Autodesk Inventor part; units mm, degrees
ref_plane "YZ Plane" through (0, 0, 0) normal (1, 0, 0) x (0, 1, 0)
ref_plane "XZ Plane" through (0, 0, 0) normal (0, 1, 0) x (-1, 0, 0)
ref_plane "XY Plane" through (0, 0, 0) normal (0, 0, 1) x (1, 0, 0)
sketch "Sketch1" plane through (0, 0, 0) normal (0, 0, 1) x (1, 0, 0)
  line L0 (-34.8609, 0) -> (34.8609, 0) construction
  line L1 (0, -34.8609) -> (0, 34.8609) construction
  line L2 (0, 0) -> (13.4339, 13.4339) construction
  line L3 (0, 0) -> (18.9985, 0) construction
  line L4 (0, 24.9006) -> (16.8, 24.9006)
  line L5 (16.8, 24.9006) -> (16.8, 21.2406)
  line L6 (16.8, 21.2406) -> (19.0203, 19.0203)
  line L7 (24.9006, 0) -> (24.9006, 16.8)
  line L8 (24.9006, 16.8) -> (21.2406, 16.8)
  line L9 (21.2406, 16.8) -> (19.0203, 19.0203)
  line L10 (0, 0) -> (-13.4339, 13.4339) construction
  line L11 (0, 0) -> (-18.9985, 0) construction
  line L12 (0, 24.9006) -> (-16.8, 24.9006)
  line L13 (-16.8, 24.9006) -> (-16.8, 21.2406)
  line L14 (-16.8, 21.2406) -> (-19.0203, 19.0203)
  line L15 (-24.9006, 0) -> (-24.9006, 16.8)
  line L16 (-24.9006, 16.8) -> (-21.2406, 16.8)
  line L17 (-21.2406, 16.8) -> (-19.0203, 19.0203)
  line L18 (0, 0) -> (13.4339, -13.4339) construction
  line L19 (0, -24.9006) -> (16.8, -24.9006)
  line L20 (16.8, -24.9006) -> (16.8, -21.2406)
  line L21 (16.8, -21.2406) -> (19.0203, -19.0203)
  line L22 (24.9006, 0) -> (24.9006, -16.8)
  line L23 (24.9006, -16.8) -> (21.2406, -16.8)
  line L24 (21.2406, -16.8) -> (19.0203, -19.0203)
  line L25 (0, 0) -> (-13.4339, -13.4339) construction
  line L26 (0, -24.9006) -> (-16.8, -24.9006)
  line L27 (-16.8, -24.9006) -> (-16.8, -21.2406)
  line L28 (-16.8, -21.2406) -> (-19.0203, -19.0203)
  line L29 (-24.9006, 0) -> (-24.9006, -16.8)
  line L30 (-24.9006, -16.8) -> (-21.2406, -16.8)
  line L31 (-21.2406, -16.8) -> (-19.0203, -19.0203)
  dimension "d0" = 45
  dimension "d1" = 3.14
  dimension "d2" = 3.66
  dimension "d3" = 16.8
extrude "Thickness" add sketch "Sketch1" along normal blind 14.9
hole "Hole1" at (0, 0, 0) direction (0, 0, 1) diameter 41.2 end through all
sketch "Sketch2" plane through (0, 0, 0) normal (0, 0, -1) x (-1, 0, 0)
  circle A0 centre (0, 0) radius 20.6
  line L0 (16.8, 24.9006) -> (-16.8, 24.9006)
  line L1 (-16.8, 24.9006) -> (-16.8, 21.2406)
  line L2 (-16.8, 21.2406) -> (-21.2406, 16.8)
  line L3 (-21.2406, 16.8) -> (-24.9006, 16.8)
  line L4 (-24.9006, 16.8) -> (-24.9006, -16.8)
  line L5 (-24.9006, -16.8) -> (-21.2406, -16.8)
  line L6 (-21.2406, -16.8) -> (-16.8, -21.2406)
  line L7 (-16.8, -21.2406) -> (-16.8, -24.9006)
  line L8 (-16.8, -24.9006) -> (16.8, -24.9006)
  line L9 (16.8, -24.9006) -> (16.8, -21.2406)
  line L10 (16.8, -21.2406) -> (21.2406, -16.8)
  line L11 (21.2406, -16.8) -> (24.9006, -16.8)
  line L12 (24.9006, -16.8) -> (24.9006, 16.8)
  line L13 (24.9006, 16.8) -> (21.2406, 16.8)
  line L14 (21.2406, 16.8) -> (16.8, 21.2406)
  line L15 (16.8, 21.2406) -> (16.8, 24.9006)
  circle A1 centre (0, 0) radius 19.6
  dimension "d17" = 1
extrude "Extrusion2" add sketch "Sketch2" against normal blind 1 contours A0
equation "\"Lens_diameter\" = 25.4"
properties part number "20_Lens_holder"
Build history of the part. All positions in model axes, mm. A direction names the side the tool comes from. Coordinates: 2 decimals unless noted, no trailing zeros. Write each loop counter-clockwise with the first axis right and the second up, starting at its lowest first coordinate (ties: lowest second). Pieces come first, ordered by that corner, then holes.
1. Band-saw the part on B-B, the plane y = 5.5. Give the cut face in (x, z), and give its area (3 significant figures).
Answer block:
outline: (-24.9, 0) - (-18.81, 0) - (-18.81, 1) - (-19.85, 1) - (-19.85, 14.9) - (-24.9, 14.9) - close; (18.81, 0) - (24.9, 0) - (24.9, 14.9) - (19.85, 14.9) - (19.85, 1) - (18.81, 1) - close
area: 153 mm2
2. Drill centre lines: probe 1 along X at (y, z) = (0, 10.5); probe 2 along Y at (x, z) = (0, 0.75). Where is each one in solid material? Low to high.
Answer block:
probe 1: x = -24.9 to -20.6, 20.6 to 24.9
probe 2: y = -24.9 to -19.6, 19.6 to 24.9
3. Drop flat-ended pins along their axis: pin 1 (1.8 mm diameter, centred on y = 24, z = 6.5, fed in from +X); pin 2 (3 mm diameter, centred on x = -22, z = 4.5, fed in from +Y); pin 3 (4 mm diameter, centred on x = -24, z = 9, fed in from -Y); pin 4 (20.5 mm diameter, centred on x = -3, y = 5, fed in from +Z). Give the stop position or say it passes through.
Answer block:
pin 1: stops at x = 16.8
pin 2: stops at y = 17.54
pin 3: stops at y = -16.8
pin 4: passes through
4. Pull direction Y, two halves, no side cores. Call faces 6 (the flat face through (-24.901, 0, 7)), 7 (the flat face through (18.99, 19.05, 7.35)), 8 (the flat face through (-11, -17, 1)): released by +Y, released by -Y, zero draft, split by the parting line, or undercut.
Answer block:
face 6: zero draft
face 7: released by +Y
face 8: undercut
5. 3-axis set-ups, long thin cutter, end or side, ignore diameter. For faces 1 (the flat face through (-16.8, -23, 7)), 2 (the flat face through (16.8, -23, 7)), 3 (the cylindrical face through (-6.19, 19.65, 8.05)), 4 (the flat face through (-16.8, 23, 7)), 5 (the flat face through (16.8, 23, 7)): which of +Z, -Z, +X, -X, +Y, -Y reach the whole face in a straight line?
Answer block:
face 1: +Z, -Z, -X, -Y
face 2: +Z, -Z, +X, -Y
face 3: +Z
face 4: +Z, -Z, -X, +Y
face 5: +Z, -Z, +X, +Y
6. Band-saw the part on A-A, the plane x = 0. Give the cut face in (y, z), and give its area (3 significant figures).
Answer block:
outline: (-24.9, 0) - (-19.6, 0) - (-19.6, 1) - (-20.6, 1) - (-20.6, 14.9) - (-24.9, 14.9) - close; (19.6, 0) - (24.9, 0) - (24.9, 14.9) - (20.6, 14.9) - (20.6, 1) - (19.6, 1) - close
area: 130 mm2
7. Band-saw the part on C-C, the plane z = 7.25. Give the cut face in (x, y), and give its area (3 significant figures).
Answer block:
outline: (-24.9, -16.8) - (-21.24, -16.8) - (-16.8, -21.24) - (-16.8, -24.9) - (16.8, -24.9) - (16.8, -21.24) - (21.24, -16.8) - (24.9, -16.8) - (24.9, 16.8) - (21.24, 16.8) - (16.8, 21.24) - (16.8, 24.9) - (-16.8, 24.9) - (-16.8, 21.24) - (-21.24, 16.8) - (-24.9, 16.8) - close; hole circle Ø41.2 at (0, 0)
area: 924 mm2
